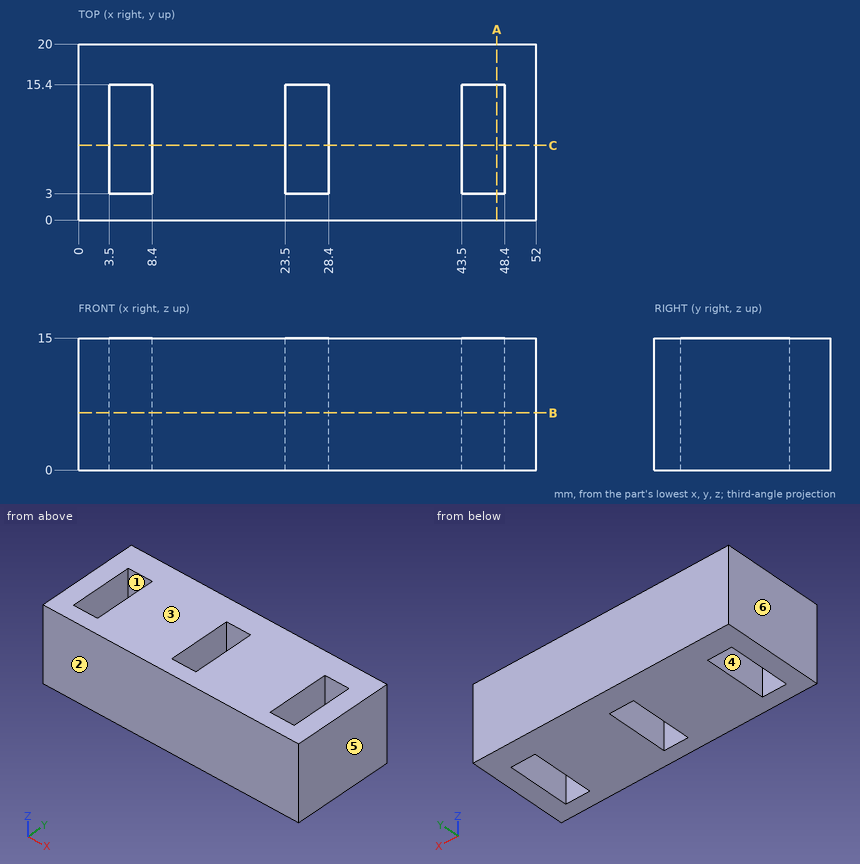
Check sheet for the drawn part. Datum: minimum x, y, z corner. Units: mm. A direction names the side the tool comes from. Round coordinates to 2 decimals unless told otherwise and drop trailing zeros. Order: outer loops, then holes, each group sorted by start corner. A loop starts at its lowest first (then second) coordinate and runs counter-clockwise, first axis right, second up.
1) Section check A-A (x = 47.5). Record the boundary of the cut face in (y, z).
2) Tool access check on the marked faces 1 and 2. Record the directions out of +Z, -Z, +X, -X, +Y, -Y that give a thin tool (end or side, any length) a straight path to the whole face; none if there is none.
3) Mould release check, pull along X, two halves, no side actions. Record for the marked faces 3, 4, 5 and 6: +X half, -X half, draft (parallel to the pull), parting line (faces both ways), or undercut.
4) Section check C-C (y = 8.5). Record the boundary of the cut face in (x, z), and give its area (4 significant figures).
5) Go/stop test with a flat-tipped pin: pin 1 Ø2.5 at (x, z) = (46, 7) entering from -Y. Record where the tip stops, or that it passes through.
6) Scan lines: line 1 (X direction, y = 8.25, z = 8.5); line 2 (Y direction, x = 45, z = 5.5). Record each from-to range of solid material in increasing order.
7) Section check B-B (z = 6.5). Record the boundary of the cut face in (x, y), and give its area (3 significant figures).
Result:
1. outline: (0, 0) - (3, 0) - (3, 15) - (0, 15) - close; (15.4, 0) - (20, 0) - (20, 15) - (15.4, 15) - close
2. face 1: +Z, -Z
2. face 2: +Z, -Z, +X, -X, -Y
3. face 3: draft
3. face 4: undercut
3. face 5: +X half
3. face 6: -X half
4. outline: (0, 0) - (3.5, 0) - (3.5, 15) - (0, 15) - close; (8.4, 0) - (23.5, 0) - (23.5, 15) - (8.4, 15) - close; (28.4, 0) - (43.5, 0) - (43.5, 15) - (28.4, 15) - close; (48.4, 0) - (52, 0) - (52, 15) - (48.4, 15) - close
4. area: 559.5 mm2
5. pin 1: stops at y = 0
6. line 1: x = 0 to 3.5, 8.4 to 23.5, 28.4 to 43.5, 48.4 to 52
6. line 2: y = 0 to 3, 15.4 to 20
7. outline: (0, 0) - (52, 0) - (52, 20) - (0, 20) - close; hole (3.5, 3) - (8.4, 3) - (8.4, 15.4) - (3.5, 15.4) - close; hole (23.5, 3) - (28.4, 3) - (28.4, 15.4) - (23.5, 15.4) - close; hole (43.5, 3) - (48.4, 3) - (48.4, 15.4) - (43.5, 15.4) - close
7. area: 858 mm2
